For this review, take the finished solid that the model builds, in its own axes (mm). Face numbers are marked on the shaded views. A direction names the side the tool comes from. Coordinates: 2 decimals unless noted, no trailing zeros. Loops run counter-clockwise (first coordinate to the right, second up) from the corner with the lowest first, then second, coordinate; pieces in that order, holes last. Notation, with made-up numbers: (2.5, 67.25) -> (31.5, 67.25) arc R28 ccw to (31.5, 97.25) -> close; hole circle Ø1 at (28, 78). An arc over 180 degrees is marked (long way). Use a Markdown table: item, result.
from build123d import *

# Parameters (mm, degrees)
SKETCH1_W           = 45
SKETCH1_H           = 50.8
SKETCH1_R           = 4
BOSS_EXTRUDE1_DEPTH = 17
FILLET1_R           = 2.54
SKETCH3_W           = 17
SKETCH3_H           = 0.254
CUT_EXTRUDE2_DEPTH  = 46
SKETCH4_W           = 12.7
SKETCH4_H           = 17
SKETCH4_R           = 2.54
BOSS_EXTRUDE2_DEPTH = 3.175


with BuildPart() as part:
    # Sketch1 → Boss-Extrude1 (new body)
    with BuildSketch(Plane.XY):
        with Locations((22.5, 25.4)):
            Rectangle(SKETCH1_W, SKETCH1_H)
        with Locations((22.4, 21)):
            Circle(SKETCH1_R, mode=Mode.SUBTRACT)
    extrude(amount=BOSS_EXTRUDE1_DEPTH)

    # Fillet1
    fillet1_edges = [part.edges().sort_by_distance(p)[0] for p in [
        (45, 0, 8.5),
        (0, 0, 8.5),
    ]]
    fillet(fillet1_edges, radius=FILLET1_R)

    # Sketch3 → Cut-Extrude2 (cut, through all)
    with BuildSketch(Plane(origin=(45, 0, 0), x_dir=(0, 0, -1), z_dir=(1, 0, 0))):
        with Locations((-8.5, 0.127)):
            Rectangle(SKETCH3_W, SKETCH3_H)
    extrude(amount=-CUT_EXTRUDE2_DEPTH, mode=Mode.SUBTRACT)

    # Sketch4 → Boss-Extrude2 (add)
    with BuildSketch(Plane(origin=(0, 50.8, 0), x_dir=(1, 0, 0), z_dir=(0, 1, 0))):
        with Locations((51.35, -8.5)):
            Rectangle(SKETCH4_W, SKETCH4_H)
        with Locations((51.35, -5.08)):
            Circle(SKETCH4_R, mode=Mode.SUBTRACT)
        with Locations((-6.35, -8.5)):
            Rectangle(SKETCH4_W, SKETCH4_H)
        with Locations((-6.35, -5.08)):
            Circle(SKETCH4_R, mode=Mode.SUBTRACT)
    extrude(amount=-BOSS_EXTRUDE2_DEPTH)


solid = part.part
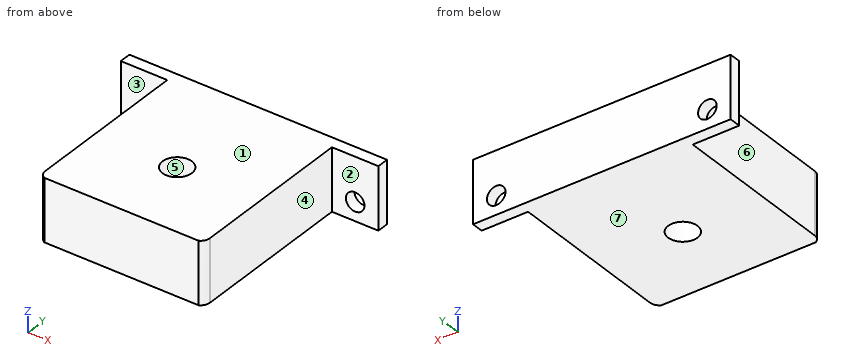
(1) Take a section at D-D on z = 15.25. Write out the cut boundary in (x, y) (3 decimals), plus the area to 3 significant figures.
Found:
| item | result |
|---|---|
| outline | (-12.7, 47.625) -> (0, 47.625) -> (0, 2.54) arc R2.54 ccw to (1.433, 0.254) -> (43.567, 0.254) arc R2.54 ccw to (45, 2.54) -> (45, 47.625) -> (57.7, 47.625) -> (57.7, 50.8) -> (-12.7, 50.8) -> close; hole circle Ø8 at (22.4, 21) |
| area | 2,300 mm^2 |
(2) Take a section at C-C on y = 21. Write out the cut boundary in (x, z), plus the area to 3 significant figures.
Found:
| item | result |
|---|---|
| outline | (0, 0) -> (18.4, 0) -> (18.4, 17) -> (0, 17) -> close; (26.4, 0) -> (45, 0) -> (45, 17) -> (26.4, 17) -> close |
| area | 629 mm^2 |
(3) For line 1 along X through (y, z) = (49.7, 5.08); line 2 along Z through (x, y) = (51.35, 50.1); line 3 along Y through (x, z) = (22.4, 4.25), list the stretches that pass through material, from the lowest coordinate up.
Found:
| item | result |
|---|---|
| line 1 | x = -12.7 to -8.89, -3.81 to 48.81, 53.89 to 57.7 |
| line 2 | z = 0 to 2.54, 7.62 to 17 |
| line 3 | y = 0.25 to 17, 25 to 50.8 |
(4) Take a section at B-B on x = 22.4. Write out the cut boundary in (y, z), plus the area to 3 significant figures.
Found:
| item | result |
|---|---|
| outline | (0.25, 0) -> (17, 0) -> (17, 17) -> (0.25, 17) -> close; (25, 0) -> (50.8, 0) -> (50.8, 17) -> (25, 17) -> close |
| area | 723 mm^2 |
(5) Mouldability with a two-part tool opening along X and no side actions: class the marked faces 4, 5, 6 and 7 as pulls with the +X half, pulls with the -X half, needs draft (parallel to the pull), parting line crosses it, or undercut.
Found:
| item | result |
|---|---|
| face 4 | pulls with the +X half |
| face 5 | undercut |
| face 6 | pulls with the -X half |
| face 7 | needs draft |
(6) For the marked faces 1, 2 and 3, list the 3-axis set-ups (+Z, -Z, +X, -X, +Y, -Y) from which the entire face can be reached by the end or side of a thin tool; tool diameter is ignored.
Found:
| item | result |
|---|---|
| face 1 | +Z, +X, -X, +Y, -Y |
| face 2 | +Z, -Z, +X, -Y |
| face 3 | +Z, -Z, -X, -Y |
(7) Take a section at A-A on z = 5.08. Write out the cut boundary in (x, y) (3 decimals).
Found:
| item | result |
|---|---|
| outline | (-12.7, 47.625) -> (-8.89, 47.625) -> (-8.89, 50.8) -> (-12.7, 50.8) -> close; (-3.81, 47.625) -> (0, 47.625) -> (0, 2.54) arc R2.54 ccw to (1.433, 0.254) -> (43.567, 0.254) arc R2.54 ccw to (45, 2.54) -> (45, 47.625) -> (48.81, 47.625) -> (48.81, 50.8) -> (-3.81, 50.8) -> close; (53.89, 47.625) -> (57.7, 47.625) -> (57.7, 50.8) -> (53.89, 50.8) -> close; hole circle Ø8 at (22.4, 21) |
(8) For pin 1 Ø4.5 at (x, z) = (51.35, 5.08) entering from -Y; pin 2 Ø1.5 at (y, z) = (14, 9) entering from -X; pin 3 Ø8.5 at (y, z) = (22.5, 6.5) entering from +X; pin 4 Ø4 at (x, z) = (-4.5, 12.5) entering from -Y (3 decimals), all flat-tipped, find the tip position at first contact; note any pin that passes through.
Found:
| item | result |
|---|---|
| pin 1 | passes through |
| pin 2 | stops at x = 0 |
| pin 3 | stops at x = 45 |
| pin 4 | stops at y = 47.625 |
